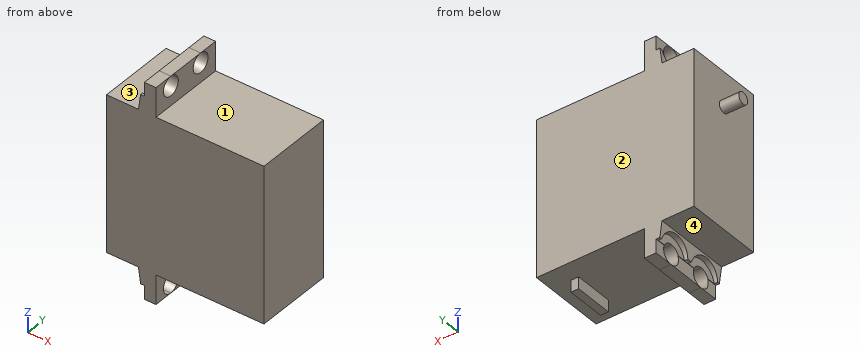
Autodesk Inventor part; units mm, degrees
ref_plane "YZ Plane" through (0, 0, 0) normal (1, 0, 0) x (0, 1, 0)
ref_plane "XZ Plane" through (0, 0, 0) normal (0, 1, 0) x (-1, 0, 0)
ref_plane "XY Plane" through (0, 0, 0) normal (0, 0, 1) x (1, 0, 0)
sketch "Sketch1" plane through (0, 0, 0) normal (0, 1, 0) x (-1, 0, 0)
  line L0 (20.2, 20) -> (-20.2, 20)
  line L1 (-20.2, 20) -> (-20.2, -20)
  line L2 (-20.2, -20) -> (20.2, -20)
  line L3 (20.2, -20) -> (20.2, 20)
  line L4 (20.2, 20) -> (-20.2, -20) construction
  line L5 (-20.2, 20) -> (20.2, -20) construction
  line L6 (-20.2, 20) -> (7.5, 20)
  line L7 (7.5, 20) -> (7.5, 27.5)
  line L8 (7.5, 27.5) -> (10.5, 27.5)
  line L9 (10.5, 27.5) -> (10.5, 20)
  line L10 (10.5, 24) -> (11.4512, 24)
  line L11 (11.4512, 24) -> (12, 20)
  line L12 (20.2, 0) -> (-20.2, 0)
  line L13 (7.5, -20) -> (7.5, -27.5)
  line L14 (7.5, -27.5) -> (10.5, -27.5)
  line L15 (10.5, -27.5) -> (10.5, -20)
  line L16 (10.5, -24) -> (11.4512, -24)
  line L17 (11.4512, -24) -> (12, -20)
  line L18 (-20.2, -20) -> (-15.2, -20)
  line L19 (-15.2, -20) -> (-15.2, -23)
  line L20 (-15.2, -23) -> (-13.2, -23)
  line L21 (-13.2, -23) -> (-13.2, -20)
  point P0 (0, 0)
  dimension "d0" = 40.4
  dimension "d1" = 40
  dimension "d2" = 27.7
  dimension "d3" = 7.5
  dimension "d4" = 3
  dimension "d5" = 5
  dimension "d6" = 2
extrude "Extrusion1" add sketch "Sketch1" along normal blind 20
sketch "Sketch3" plane through (-20.2, 0, -20) normal (-1, 0, 0) x (0, 0, 1)
  circle A0 centre (31, 10) radius 1.5
  line L0 (47.5, 0) -> (47.5, 20)
  line L1 (47.5, 10) -> (-7.5, 10)
  line L2 (-7.5, 0) -> (-7.5, 20)
  line L3 (20, 0) -> (20, 20)
  line L4 (0, 20) -> (40, 20)
  circle A1 centre (45, 5) radius 2.5
  circle A2 centre (45, 15) radius 2.5
  circle A3 centre (-5, 5) radius 2.5
  circle A4 centre (-5, 15) radius 2.5
  line L5 (45, 5) -> (45, 5)
  dimension "d24" = 0
sketch "Sketch4" plane through (15.2, 0, -23) normal (0, 0, -1) x (-1, 0, 0)
  line L0 (0, 0) -> (0, 20)
  line L1 (4, 25) -> (0, 25)
  line L2 (0, 25) -> (0, 15)
  line L3 (0, 15) -> (4, 15)
  line L4 (4, 15) -> (4, 25)
  line L5 (2, 0) -> (2, 20)
  line L6 (4, 25) -> (0, 15) construction
  line L7 (0, 25) -> (4, 15) construction
  line L8 (4, -5) -> (0, -5)
  line L9 (0, -5) -> (0, 5)
  line L10 (0, 5) -> (4, 5)
  line L11 (4, 5) -> (4, -5)
  line L12 (4, -5) -> (0, 5) construction
  line L13 (0, -5) -> (4, 5) construction
  point P0 (15.2, 0)
extrude "Extrusion4" cut sketch "Sketch4" against normal blind 3 contours L0 L10 L11 L8 L9 | L0 L2 L1 L4 L3
extrude "Extrusion5" cut sketch "Sketch3" against normal blind 15 contours A3 | A4 | A2 | A1
extrude "Extrusion6" add sketch "Sketch3" along normal blind 5 contours L1 A0 | A0 L1
thread "Thread1"
thread "Thread2"
thread "Thread3"
thread "Thread4"
sketch "Sketch5" plane through (-20.2, 0, -20) normal (-1, 0, 0) x (0, 0, 1)
  circle A0 centre (45, 15) radius 4.5
  circle A1 centre (45, 5) radius 4.5
  circle A2 centre (-5, 5) radius 2.5
  circle A3 centre (-5, 5) radius 4.5
  circle A4 centre (-5, 15) radius 2.5
  circle A5 centre (-5, 15) radius 4.5
  point P0 (20, 0)
  point P1 (-7.5, 5)
  point P2 (-7.5, 15)
  dimension "d33" = 9
  dimension "d34" = 9
  dimension "d35" = 9
  dimension "d36" = 9
extrude "Extrusion7" cut sketch "Sketch5" against normal blind 9.6 contours A0 | A1 | A2 | A3 | A5
properties part number "Servo"
Source: CAD feature listing. Evaluate the final solid. Frame: model axes, mm. Face numbers are marked on the shaded views. A direction names the side the tool comes from. Coordinates: 2 decimals unless noted, no trailing zeros. Loops run counter-clockwise (first coordinate to the right, second up) from the corner with the lowest first, then second, coordinate; pieces in that order, holes last. Notation, with made-up numbers: (-21.5, 0.5) - (23.5, 0.5) arc R25 cw to (23.5, 24.5) - close; hole circle Ø11 at (-9, 87). An arc over 180 degrees is marked (long way). Answer as CSV lines item,"result".
1. Reachability of the marked faces 1, 2, 3 and 4 from +Z, -Z, +X, -X, +Y, -Y: full face, straight path, thin tool, end or side. Return the list, or none.
Established:
face 1,"+Z, +X, +Y, -Y"
face 2,"+Z, -Z, +X, -X, +Y"
face 3,"+Z, -X, +Y, -Y"
face 4,"-Z, -X, +Y, -Y"
2. Ray query, line 1 (Y direction, x = -9, z = 25); line 2 (Z direction, x = -16.5, y = 13); line 3 (X direction, y = 2.5, z = -2.5). Return the intervals inside material, ascending.
Established:
line 1,"y = 0 to 2.5, 7.5 to 12.5, 17.5 to 20"
line 2,"z = -20 to 20"
line 3,"x = -20.2 to 20.2"
3. Section A-A (y = 13.75). Return loops of the section in (x, z), then the cut area to 3 significant figures.
Established:
outline,"(-20.2, -20) - (-12, -20) - (-11.91, -20.68) - (-10.6, -20.68) - (-10.6, -22.83) - (-7.5, -22.83) - (-7.5, -20) - (13.2, -20) - (13.2, -23) - (15.2, -23) - (15.2, -20) - (20.2, -20) - (20.2, 20) - (-7.5, 20) - (-7.5, 22.83) - (-10.6, 22.83) - (-10.6, 20.68) - (-11.91, 20.68) - (-12, 20) - (-20.2, 20) - close; (-10.5, -27.5) - (-7.5, -27.5) - (-7.5, -27.17) - (-10.5, -27.17) - close; (-10.5, 27.17) - (-7.5, 27.17) - (-7.5, 27.5) - (-10.5, 27.5) - close"
area,"1,640 mm2"
4. Contact query for flat-ended pins moving along their axis: pin 1 (3 mm diameter, centred on x = -20.5, y = 17.5, fed in from +Z); pin 2 (1.8 mm diameter, centred on y = 15, z = -22.5, fed in from -X); pin 3 (0.8 mm diameter, centred on x = -11, y = 10, fed in from +Z). Output: stop coordinate, or through.
Established:
pin 1,"stops at z = 20"
pin 2,"stops at x = -10.6"
pin 3,"stops at z = 24"
5. Section C-C (y = 10). Return loops of the section in (x, z).
Established:
outline,"(-25.2, 9.5) - (-20.2, 9.5) - (-20.2, -20) - (-12, -20) - (-11.45, -24) - (-10.5, -24) - (-10.5, -27.5) - (-7.5, -27.5) - (-7.5, -20) - (13.2, -20) - (13.2, -23) - (15.2, -23) - (15.2, -20) - (20.2, -20) - (20.2, 20) - (-7.5, 20) - (-7.5, 27.5) - (-10.5, 27.5) - (-10.5, 24) - (-11.45, 24) - (-12, 20) - (-20.2, 20) - (-20.2, 12.5) - (-25.2, 12.5) - close"
6. Section D-D (z = 11). Return loops of the section in (x, y), then the cut area to 3 significant figures.
Established:
outline,"(-25.2, 8.5) - (-20.2, 8.5) - (-20.2, 0) - (20.2, 0) - (20.2, 20) - (-20.2, 20) - (-20.2, 11.5) - (-25.2, 11.5) - close"
area,"823 mm2"
7. Section B-B (z = 25). Return loops of the section in (x, y), then the cut area to 3 significant figures.
Established:
outline,"(-10.5, 0) - (-7.5, 0) - (-7.5, 2.5) - (-10.5, 2.5) - close; (-10.5, 7.5) - (-7.5, 7.5) - (-7.5, 12.5) - (-10.5, 12.5) - close; (-10.5, 17.5) - (-7.5, 17.5) - (-7.5, 20) - (-10.5, 20) - close"
area,"30.0 mm2"
